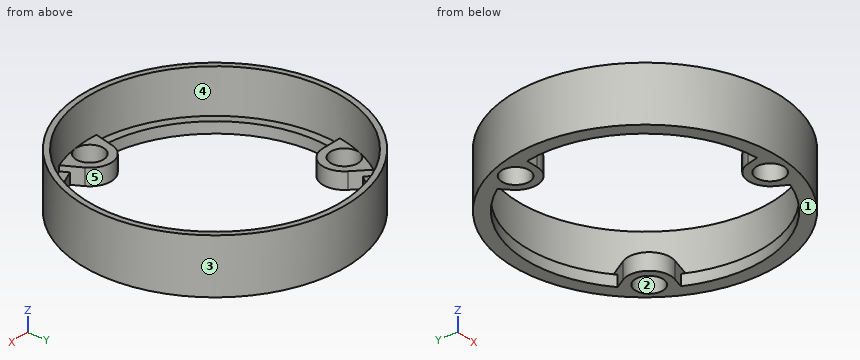
from build123d import *

# Parameters (mm, degrees)
SKETCH001_R        = 2.625
POCKET_DEPTH       = 5.5
PAD_DEPTH          = 3
POLARPATTERN_COUNT = 3
SKETCH002_R        = 2.5
POCKET001_DEPTH    = 13.001


with BuildPart() as part:
    # Sketch → Revolution (revolve)
    with BuildSketch(Plane.XZ):
        Polygon((21.5, 5), (21.5, 3), (24, 3), (24, 13), (23, 13), (23, 5), align=None)
    revolve(axis=Axis((0, 0, 0), (0, 0, 1)))

    # Sketch001 → Pocket (cut)
    with BuildSketch(Plane.XY):
        with Locations((-17.5, 0)):
            Circle(SKETCH001_R)
        with Locations((-8.75, 15.1554445662)):
            Circle(SKETCH001_R)
        with Locations((8.75, 15.1554445662)):
            Circle(SKETCH001_R)
        with Locations((17.5, 0)):
            Circle(SKETCH001_R)
        with Locations((8.75, -15.1554445662)):
            Circle(SKETCH001_R)
        with Locations((-8.75, -15.1554445662)):
            Circle(SKETCH001_R)
    extrude(amount=POCKET_DEPTH, mode=Mode.SUBTRACT)

    # Sketch003 → Pad (join)
    with BuildSketch(Plane.XY.offset(3)):
        with BuildLine():
            ThreePointArc((-19.0869375712, 12.8331139694), (-21.405483769, 8.4145864197), (-22.716513817, 3.6))
            Line((-19.0788007507, 3.6), (-22.716513817, 3.6))
            ThreePointArc((-19.0788007507, 3.6), (-15.4492148319, 6.0731518485), (-16.4230212393, 10.3559167367))
            Line((-16.4230212393, 10.3559167367), (-19.0869375712, 12.8331139694))
        make_face()
    pad = extrude(amount=PAD_DEPTH)

    # PolarPattern: Pad ×3 about axis
    polarpattern_axis = Axis((0, 0, 3), (0, 0, 1))
    for i in range(1, POLARPATTERN_COUNT):
        add(pad.rotate(polarpattern_axis, i * 360 / POLARPATTERN_COUNT))

    # Sketch002 → Pocket001 (cut, through all)
    with BuildSketch(Plane.XY):
        with Locations((16.0345540639, 12.7727473933)):
            Circle(SKETCH002_R)
        with Locations((3.0442466868, -20.2727048543)):
            Circle(SKETCH002_R)
        with Locations((-19.0788007507, 7.499957461)):
            Circle(SKETCH002_R)
    extrude(amount=POCKET001_DEPTH, mode=Mode.SUBTRACT)


solid = part.part
The model under review builds one solid part; all positions refer to its coordinate system, in mm. Face numbers are marked on the shaded views. A direction names the side the tool comes from. Round coordinates to 2 decimals unless told otherwise and drop trailing zeros. Loops run counter-clockwise (first coordinate to the right, second up) from the corner with the lowest first, then second, coordinate; pieces in that order, holes last. Notation, with made-up numbers: (2.25, 8.5) -> (43.25, 8.5) arc R21 ccw to (43.25, 29.5) -> close; hole circle Ø3 at (-13, 66). An arc over 180 degrees is marked (long way). Write item = value, one per line. Start each with the question number.
Item 1: Insertion check: pin 1 (1.5 mm diameter, centred on y = -15, z = 6.5, fed in from -X); pin 2 (3.5 mm diameter, centred on x = -21, z = 5, fed in from -Y); pin 3 (11 mm diameter, centred on x = -16, y = -3.5, fed in from +Z); pin 4 (6 mm diameter, centred on x = -19.08, y = 7.5, fed in from -Z). Each pin has a flat end and moves straight along its axis. Give the tip position at first contact, or say it passes through.
Item 2: Take a section at C-C on z = 4. Give the boundary of the cut face in (x, y).
Item 3: Take a section at D-D on x = -2.5. Give the boundary of the cut face in (y, z), plus the area to 3 significant figures.
Item 4: Take a section at B-B on x = 4.5. Give the boundary of the cut face in (y, z).
Item 5: Mouldability with a two-part tool opening along X and no side actions: class the marked faces 1, 2 and 3 as released by +X, released by -X, zero draft, split by the parting line, or undercut.
Item 6: For the marked faces 4 and 5, list the 3-axis set-ups (+Z, -Z, +X, -X, +Y, -Y) from which the entire face can be reached by the end or side of a thin tool; tool diameter is ignored.
Item 7: Take a section at A-A on y = 0. Give the boundary of the cut face in (x, z), plus the area to 3 significant figures.
Item 8: To check wall thickness, follow L1, parallel to X at y = -19.5, z = 4; L2, parallel to X at y = -17.5, z = 4; L3, parallel to Y at x = 5.5, z = 9.5. State the ranges of each line that lie inside material, in increasing order.
Result:
q1.pin_1 = -19.31
q1.pin_2 = -14.33
q1.pin_3 = 5
q1.pin_4 = 3
q2.outline = circle Ø48 at (0, 0); hole circle Ø5 at (-19.08, 7.5); hole (-21.2, 3.6) arc R21.5 ccw to (-1.23, -21.46) -> (-0.76, -19.4) arc R3.9 cw to (6.42, -18.32) -> (7.48, -20.16) arc R21.5 ccw to (19.2, 9.67) -> (17.18, 9.04) arc R3.9 cw to (12.66, 14.72) -> (13.72, 16.56) arc R21.5 ccw to (-17.97, 11.8) -> (-16.42, 10.36) arc R3.9 cw to (-19.08, 3.6) -> close; hole circle Ø5 at (3.04, -20.27); hole circle Ø5 at (16.03, 12.77)
q3.outline = (-23.87, 3) -> (-21.35, 3) -> (-21.35, 5) -> (-22.86, 5) -> (-22.86, 13) -> (-23.87, 13) -> close; (21.35, 3) -> (23.87, 3) -> (23.87, 13) -> (22.86, 13) -> (22.86, 5) -> (21.35, 5) -> close
q3.area = 26.2 mm²
q4.outline = (-23.57, 3) -> (-22.31, 3) -> (-22.31, 6) -> (-22.56, 6) -> (-22.56, 13) -> (-23.57, 13) -> close; (-18.24, 3) -> (-16.65, 3) -> (-16.65, 6) -> (-18.24, 6) -> close; (21.02, 3) -> (23.57, 3) -> (23.57, 13) -> (22.56, 13) -> (22.56, 5) -> (21.02, 5) -> close
q5.face_1 = zero draft
q5.face_2 = undercut
q5.face_3 = split by the parting line
q6.face_4 = +Z
q6.face_5 = +Z, -Z
q7.outline = (-24, 3) -> (-21.5, 3) -> (-21.5, 5) -> (-23, 5) -> (-23, 13) -> (-24, 13) -> close; (21.5, 3) -> (24, 3) -> (24, 13) -> (23, 13) -> (23, 5) -> (21.5, 5) -> close
q7.area = 26.0 mm²
q8.L1 = -13.99 to -9.06, -0.78 to 0.67, 5.42 to 7.1, 9.06 to 13.99
q8.L2 = -16.42 to -12.49, 0.3 to 5.79, 12.49 to 16.42
q8.L3 = -23.36 to -22.33, 22.33 to 23.36
